Build history of the part. All positions in model axes, mm. A direction names the side the tool comes from. Round coordinates to 2 decimals unless told otherwise and drop trailing zeros. Write each loop counter-clockwise with the first axis right and the second up, starting at its lowest first coordinate (ties: lowest second). Pieces come first, ordered by that corner, then holes. Notation, with made-up numbers: (24.5, 77.5) -> (44.5, 77.5) arc R7 ccw to (44.5, 81.5) -> close; hole circle Ø9 at (38.5, 9). An arc over 180 degrees is marked (long way). Answer in a Markdown table with one row per item.
```python
from build123d import *

# Parameters (mm, degrees)
SKETCH1_W               = 101.219
SKETCH1_H               = 112.141
BOSS_EXTRUDE1_DEPTH     = 1.27
SKETCH2_W               = 53.34
SKETCH2_H               = 101.981
BOSS_EXTRUDE2_DEPTH     = 15.24
SKETCH3_W               = 76.2
SKETCH3_H               = 50.8
BOSS_EXTRUDE3_DEPTH     = 21.59
CUT_EXTRUDE1_DEPTH      = 79.916424529
CUT_EXTRUDE1_DEPTH_BACK = 79.916424529
SKETCH4_R               = 1.27


with BuildPart() as part:
    # Sketch1 → Boss-Extrude1 (new body)
    with BuildSketch(Plane.XY):
        Rectangle(SKETCH1_W, SKETCH1_H)
    extrude(amount=BOSS_EXTRUDE1_DEPTH)

    # Sketch2 → Boss-Extrude2 (add)
    with BuildSketch(Plane.XY.offset(1.27)):
        with Locations((-4.8895, 0)):
            Rectangle(SKETCH2_W, SKETCH2_H)
    extrude(amount=BOSS_EXTRUDE2_DEPTH)

    # Sketch3 → Boss-Extrude3 (add)
    with BuildSketch(Plane(origin=(0, 0, 0), x_dir=(-1, 0, 0), z_dir=(0, 0, -1))):
        with Locations((-3.6195, 11.6205)):
            Rectangle(SKETCH3_W, SKETCH3_H)
    extrude(amount=BOSS_EXTRUDE3_DEPTH)

    # Sketch4 → Cut-Extrude1 (cut, two sides: drawn at the far end of the back side and taken through both)
    with BuildSketch(Plane.XY.offset(1.27).offset(-CUT_EXTRUDE1_DEPTH_BACK)):
        with Locations(Location((-29.6545, 52.7685, 0), (0, 0, 180))):
            Circle(SKETCH4_R)
        with Locations(Location((19.8755, 52.7685, 0), (0, 0, 180))):
            Circle(SKETCH4_R)
        with Locations(Location((-29.6545, -52.7685, 0), (0, 0, 180))):
            Circle(SKETCH4_R)
        with Locations(Location((19.8755, -52.7685, 0), (0, 0, 180))):
            Circle(SKETCH4_R)
    extrude(amount=CUT_EXTRUDE1_DEPTH + CUT_EXTRUDE1_DEPTH_BACK, mode=Mode.SUBTRACT)


solid = part.part
```
Q1. Saw through at A-A on y = -10. Write the cut outline in (x, z), plus the area to 3 significant figures.
A:
| item | result |
|---|---|
| outline | (-50.61, 0) -> (-34.48, 0) -> (-34.48, -21.59) -> (41.72, -21.59) -> (41.72, 0) -> (50.61, 0) -> (50.61, 1.27) -> (21.78, 1.27) -> (21.78, 16.51) -> (-31.56, 16.51) -> (-31.56, 1.27) -> (-50.61, 1.27) -> close |
| area | 2,590 mm² |
Q2. Which spindle directions (+Z, -Z, +X, -X, +Y, -Y) get a long thin tool onto all of the face, cutting with end or side? Do faces 1 (the flat face through (-5, 50.99, 9)), 2 (the flat face through (41.72, 11, -11)), 3 (the flat face through (-5, -50.99, 9)), 4 (the flat face through (-34.48, 11, -11)), 5 (the flat face through (4, -13.779, -11)). Say none if no direction does.
A:
| item | result |
|---|---|
| face 1 | +Z, +X, -X, +Y |
| face 2 | -Z, +X, +Y, -Y |
| face 3 | +Z, +X, -X, -Y |
| face 4 | -Z, -X, +Y, -Y |
| face 5 | -Z, +X, -X, -Y |
Q3. Drop flat-ended pins along their axis: P1, Ø5, axis at x = -3.5, z = -10.5, coming from the -Y side; P2, Ø2, axis at x = -29.65, y = -52.77, coming from the +Z side; P3, Ø2, axis at x = 15, z = 6, coming from the -Y side; P4, Ø6.5, axis at y = 1, z = -12.5, coming from the +X side. Give the stop position or say it passes through.
A:
| item | result |
|---|---|
| P1 | y = -13.78 |
| P2 | through |
| P3 | y = -50.99 |
| P4 | x = 41.72 |
Q4. Two-plate mould, pull along X, no slides. Class faces 6 (the cylindrical face through (20.15, -51.53, 0.63)), 7 (the flat face through (-31.56, -1, 9)), 8 (the flat face through (-5, 1, 16.51)): released by +X, released by -X, zero draft, split by the parting line, or undercut.
A:
| item | result |
|---|---|
| face 6 | undercut |
| face 7 | released by -X |
| face 8 | zero draft |
Q5. Saw through at B-B on x = -9. Write the cut outline in (y, z), plus the area to 3 significant figures.
A:
| item | result |
|---|---|
| outline | (-56.07, 0) -> (-13.78, 0) -> (-13.78, -21.59) -> (37.02, -21.59) -> (37.02, 0) -> (56.07, 0) -> (56.07, 1.27) -> (50.99, 1.27) -> (50.99, 16.51) -> (-50.99, 16.51) -> (-50.99, 1.27) -> (-56.07, 1.27) -> close |
| area | 2,790 mm² |
Q6. Saw through at D-D on y = -28.5. Write the cut outline in (x, z), plus the area to 3 significant figures.
A:
| item | result |
|---|---|
| outline | (-50.61, 0) -> (50.61, 0) -> (50.61, 1.27) -> (21.78, 1.27) -> (21.78, 16.51) -> (-31.56, 16.51) -> (-31.56, 1.27) -> (-50.61, 1.27) -> close |
| area | 941 mm² |
Q7. Saw through at C-C on z = -15. Write the cut outline in (x, y).
A:
| item | result |
|---|---|
| outline | (-34.48, -13.78) -> (41.72, -13.78) -> (41.72, 37.02) -> (-34.48, 37.02) -> close |
Q8. Wall check: line 1 (Z direction, x = 34.5, y = -42); line 2 (X direction, y = 32, z = -1.5); line 3 (Z direction, x = 9, y = -25). Give the ranges that are in metal, low to high. Write a range as [from, to].
A:
| item | result |
|---|---|
| line 1 | [0, 1.27] |
| line 2 | [-34.48, 41.72] |
| line 3 | [0, 16.51] |
